For this review, use the dimensioned drawing (mm, ordinates from the lowest corner) and the shaded views. Coordinates: 2 decimals unless noted, no trailing zeros. Loops run counter-clockwise (first coordinate to the right, second up) from the corner with the lowest first, then second, coordinate; pieces in that order, holes last. Notation, with made-up numbers: (-10.5, 13.5) - (-3.5, 13.5) arc R18 ccw to (-3.5, 39.5) - close; hole circle Ø8 at (60.25, 59). An arc over 180 degrees is marked (long way). Answer in a Markdown table with one row per item. Add a question column.
(1) We need section A-A, the plane y = 4. Write out the cut boundary in (x, z).
(2) We need section B-B, the plane x = 31. Write out the cut boundary in (y, z).
(3) Clearance check with a flat-ended pin moving along its axis: pin 1 (1.7 mm diameter, centred on x = 31, y = 4, fed in from +Z). State where the tip first meets the part, or that it passes through.
(4) To check wall thickness, follow L1, parallel to Y at x = 4, z = 0.6; L2, parallel to X at y = 75, z = 0.8; L3, parallel to Y at x = 4.5, z = 0.9. State the ranges of each line that lie inside material, in increasing order. Write a range as [from, to].
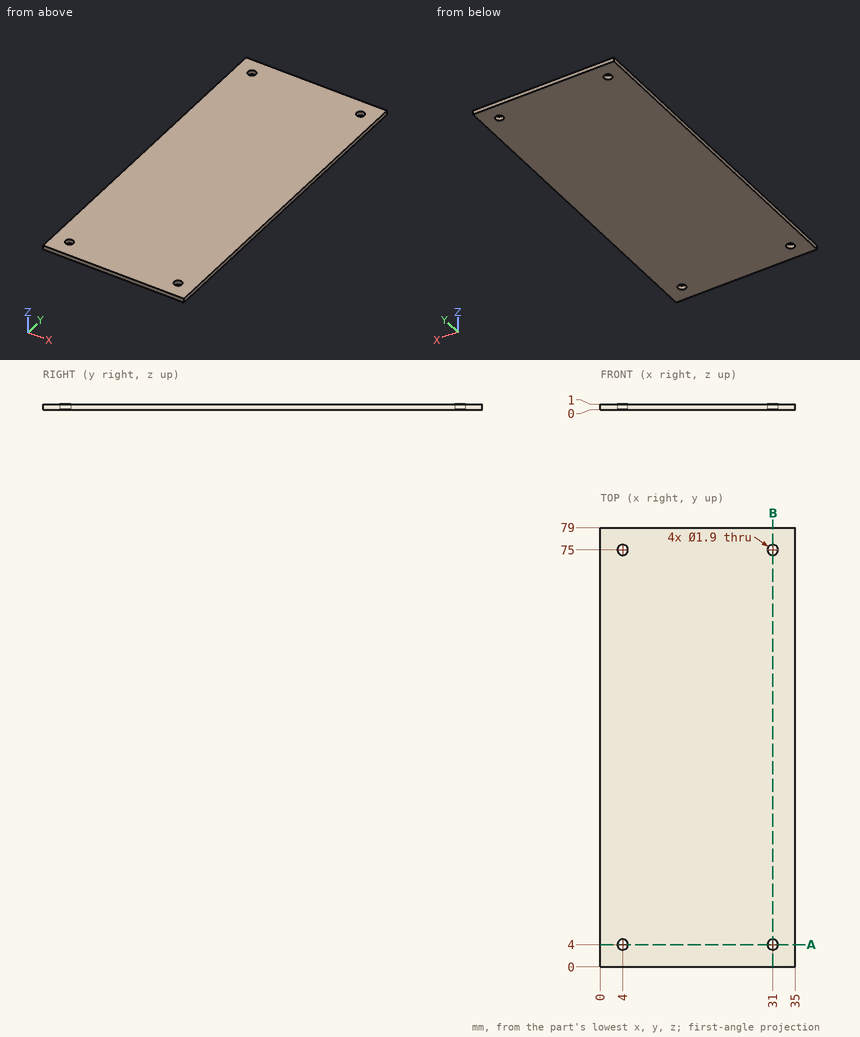
Responses:
| question | item | result |
|---|---|---|
| 1 | outline | (0, 0) - (3.05, 0) - (3.05, 1) - (0, 1) - close; (4.95, 0) - (30.05, 0) - (30.05, 1) - (4.95, 1) - close; (31.95, 0) - (35, 0) - (35, 1) - (31.95, 1) - close |
| 2 | outline | (0, 0) - (3.05, 0) - (3.05, 1) - (0, 1) - close; (4.95, 0) - (74.05, 0) - (74.05, 1) - (4.95, 1) - close; (75.95, 0) - (79, 0) - (79, 1) - (75.95, 1) - close |
| 3 | pin 1 | passes through |
| 4 | L1 | y = [0, 3.05], [4.95, 74.05], [75.95, 79] |
| 4 | L2 | x = [0, 3.05], [4.95, 30.05], [31.95, 35] |
| 4 | L3 | y = [0, 3.19], [4.81, 74.19], [75.81, 79] |
